The listing builds one solid part. Answer for the finished solid, in the listing's coordinates (mm). Face numbers are marked on the shaded views. A direction names the side the tool comes from. Coordinates: 2 decimals unless noted, no trailing zeros. Order: outer loops, then holes, each group sorted by start corner. A loop starts at its lowest first (then second) coordinate and runs counter-clockwise, first axis right, second up. Notation, with made-up numbers: (37, -9.5) -> (78, -9.5) arc R6 ccw to (78, 0.5) -> close; hole circle Ø8 at (-2, -28.75). An arc over 180 degrees is marked (long way). Return JSON: item names as keys, results as strings.
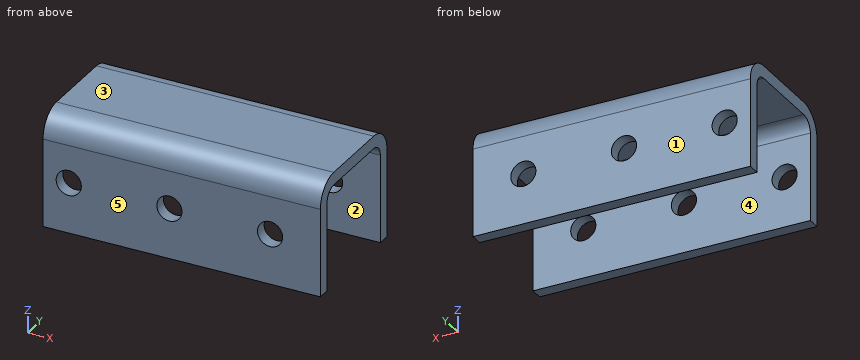
```python
from build123d import *

# Parameters (mm, degrees)
SKETCH1_W          = 889
SKETCH1_H          = 31.75
EXTRUDE1_DEPTH     = 28.575
EXTRUDE2_REACH     = 891
SKETCH2_W          = 25.4
SKETCH2_H          = 25.4
HOLE1_D            = 6.35
HOLE1_DEPTH        = 3.175
LPATTERN1_COUNT    = 35
LPATTERN1_PITCH    = 25.4
HOLE2_D            = 9.652
HOLE2_DEPTH        = 3.175
LPATTERN2_COUNT    = 12
LPATTERN2_PITCH    = 25.4
HOLE3_D            = 9.652
HOLE3_DEPTH        = 3.175
HOLE4_D            = 9.652
HOLE4_DEPTH        = 3.175
LPATTERN3_COUNT    = 12
LPATTERN3_PITCH    = 25.4
HOLE5_D            = 3.175
HOLE5_DEPTH        = 3.175
HOLE6_D            = 6.35
HOLE6_DEPTH        = 3.175
LPATTERN4_COUNT    = 35
LPATTERN4_PITCH    = 25.4
FILLET1_R          = 3.175
FILLET2_R          = 3.175
FILLET3_R          = 6.35
FILLET4_R          = 6.35
SKETCH16_W         = 145.760071232
SKETCH16_H         = 71.504803879
CUT_EXTRUDE2_DEPTH = 75
SKETCH17_W         = 473.628565651
SKETCH17_H         = 66.908943447
CUT_EXTRUDE3_DEPTH = 186
SKETCH18_W         = 373.094897193
SKETCH18_H         = 93.915816603
CUT_EXTRUDE4_DEPTH = 186


with BuildPart() as part:
    # Sketch1 → Extrude1 (new body)
    with BuildSketch(Plane.XY.offset(3.175)):
        with Locations((428.480011997, 8.672957166)):
            Rectangle(SKETCH1_W, SKETCH1_H)
    extrude(amount=-EXTRUDE1_DEPTH)

    # Sketch2 → Extrude2 (cut, up to next)
    with BuildSketch(Plane.ZY.offset(16.019988003), mode=Mode.PRIVATE) as extrude2_sk1:
        with Locations((-12.7, 8.672957166)):
            Rectangle(SKETCH2_W, SKETCH2_H)
    extrude2_tool1 = extrude(extrude2_sk1.sketch, amount=-EXTRUDE2_REACH, mode=Mode.PRIVATE) & part.part
    add(extrude2_tool1.solids().sort_by_distance((-16.019988, 8.672957, -12.7))[0], mode=Mode.SUBTRACT)

    # Hole1
    with Locations(Plane(origin=(0, 24.547957166, 0), x_dir=(-1, 0, 0), z_dir=(0, 1, 0))):
        with Locations((3.319988003, -12.7)):
            hole1 = Hole(HOLE1_D / 2, depth=HOLE1_DEPTH)

    # LPattern1: Hole1 ×35
    with Locations(*[(i * LPATTERN1_PITCH, 0, 0) for i in range(1, LPATTERN1_COUNT)]):
        add(hole1, mode=Mode.SUBTRACT)

    # Hole2
    with Locations(Plane.XY.offset(3.175)):
        with Locations((66.530011997, 10.577957166)):
            hole2 = Hole(HOLE2_D / 2, depth=HOLE2_DEPTH)

    # LPattern2: Hole2 ×12, 8 skipped
    with Locations(*[(i * LPATTERN2_PITCH, 0, 0) for i in range(1, LPATTERN2_COUNT) if i not in (2, 3, 4, 5, 6, 7, 8, 9)]):
        add(hole2, mode=Mode.SUBTRACT)

    # Hole3
    with Locations(Plane.XY.offset(3.175)):
        with Locations((428.480011997, 6.767957166)):
            Hole(HOLE3_D / 2, depth=HOLE3_DEPTH)

    # Hole4
    with Locations(Plane.XY.offset(3.175)):
        with Locations((511.030011997, 10.577957166)):
            hole4 = Hole(HOLE4_D / 2, depth=HOLE4_DEPTH)

    # LPattern3: Hole4 ×12, 8 skipped
    with Locations(*[(i * LPATTERN3_PITCH, 0, 0) for i in range(1, LPATTERN3_COUNT) if i not in (2, 3, 4, 5, 6, 7, 8, 9)]):
        add(hole4, mode=Mode.SUBTRACT)

    # Hole5
    with Locations(Plane.XY.offset(3.175)):
        with Locations((669.780011997, 8.672957166)):
            Hole(HOLE5_D / 2, depth=HOLE5_DEPTH)

    # Hole6
    with Locations(Plane(origin=(0, -4.027042834, 0), x_dir=(-1, 0, 0), z_dir=(0, 1, 0))):
        with Locations((3.319988003, -12.7)):
            hole6 = Hole(HOLE6_D / 2, depth=HOLE6_DEPTH)

    # LPattern4: Hole6 ×35
    with Locations(*[(i * LPATTERN4_PITCH, 0, 0) for i in range(1, LPATTERN4_COUNT)]):
        add(hole6, mode=Mode.SUBTRACT)

    # Fillet1
    fillet1_edges = [part.edges().sort_by_distance(p)[0] for p in [
        (428.480011997, 21.372957166, 0),
    ]]
    fillet(fillet1_edges, radius=FILLET1_R)

    # Fillet2
    fillet2_edges = [part.edges().sort_by_distance(p)[0] for p in [
        (428.480011997, -4.027042834, 0),
    ]]
    fillet(fillet2_edges, radius=FILLET2_R)

    # Fillet3
    fillet3_edges = [part.edges().sort_by_distance(p)[0] for p in [
        (428.480011997, -7.202042834, 3.175),
    ]]
    fillet(fillet3_edges, radius=FILLET3_R)

    # Fillet4
    fillet4_edges = [part.edges().sort_by_distance(p)[0] for p in [
        (428.480011997, 24.547957166, 3.175),
    ]]
    fillet(fillet4_edges, radius=FILLET4_R)

    # Sketch16 → Cut-Extrude2 (cut)
    with BuildSketch(Plane(origin=(0, 24.547957166, 0), x_dir=(1, 0, 0), z_dir=(0, 1, 0))):
        with Locations((40.099976381, -10.352401939)):
            Rectangle(SKETCH16_W, SKETCH16_H)
    extrude(amount=-CUT_EXTRUDE2_DEPTH, mode=Mode.SUBTRACT)

    # Sketch17 → Cut-Extrude3 (cut)
    with BuildSketch(Plane(origin=(0, 24.547957166, 0), x_dir=(1, 0, 0), z_dir=(0, 1, 0))):
        with Locations((288.165729172, -8.054471723)):
            Rectangle(SKETCH17_W, SKETCH17_H)
    extrude(amount=-CUT_EXTRUDE3_DEPTH, mode=Mode.SUBTRACT)

    # Sketch18 → Cut-Extrude4 (cut)
    with BuildSketch(Plane(origin=(0, 24.547957166, 0), x_dir=(1, 0, 0), z_dir=(0, 1, 0))):
        with Locations((616.432563401, -21.557908301)):
            Rectangle(SKETCH18_W, SKETCH18_H)
    extrude(amount=-CUT_EXTRUDE4_DEPTH, mode=Mode.SUBTRACT)


solid = part.part
```
Item 1: Determine the mould class of the marked faces 1, 2 and 3 for opening direction Y: pulls with the +Y half, pulls with the -Y half, needs draft (parallel to the pull), parting line crosses it, or undercut.
Answer list:
{"face 1": "pulls with the +Y half", "face 2": "undercut", "face 3": "needs draft"}
Item 2: Which of the six approach directions +Z, -Z, +X, -X, +Y, -Y give full straight-line access (tool end or side, diameter ignored) to the marked faces 4 and 5?
Answer list:
{"face 4": "-Z, +X, -X", "face 5": "+Z, -Z, +X, -X, -Y"}
Item 3: The part is cut by section B-B on z = -12.7. Count the separate pieces of the cut face and the enclosed holes in it, plus the area to 3 significant figures.
Answer list:
{"separate pieces": "8", "enclosed holes": "0", "area": "324 mm2"}
Item 4: The part is cut by section D-D on x = 861.5. Determine the outline of the cut face in (y, z) (3 decimals).
Answer list:
{"outline": "(-7.202, -25.4) -> (-4.027, -25.4) -> (-4.027, -15.631) -> (-7.202, -15.631) -> close; (-7.202, -9.769) -> (-4.027, -9.769) -> (-4.027, -3.175) arc R3.175 cw to (-0.852, 0) -> (18.198, 0) arc R3.175 cw to (21.373, -3.175) -> (21.373, -9.769) -> (24.548, -9.769) -> (24.548, -3.175) arc R6.35 ccw to (18.198, 3.175) -> (-0.852, 3.175) arc R6.35 ccw to (-7.202, -3.175) -> close; (21.373, -25.4) -> (24.548, -25.4) -> (24.548, -15.631) -> (21.373, -15.631) -> close"}
Item 5: The part is cut by section C-C on y = 4.5. Determine the outline of the cut face in (x, z) (3 decimals), plus the area to 3 significant figures.
Answer list:
{"outline": "(802.98, 0) -> (872.98, 0) -> (872.98, 3.175) -> (802.98, 3.175) -> close", "area": "222 mm2"}
Item 6: The part is cut by section A-A on x = 810.5. Determine the outline of the cut face in (y, z) (3 decimals), plus the area to 3 significant figures.
Answer list:
{"outline": "(-7.202, -25.4) -> (-4.027, -25.4) -> (-4.027, -15.707) -> (-7.202, -15.707) -> close; (-7.202, -9.693) -> (-4.027, -9.693) -> (-4.027, -3.175) arc R3.175 cw to (-0.852, 0) -> (18.198, 0) arc R3.175 cw to (21.373, -3.175) -> (21.373, -9.693) -> (24.548, -9.693) -> (24.548, -3.175) arc R6.35 ccw to (18.198, 3.175) -> (-0.852, 3.175) arc R6.35 ccw to (-7.202, -3.175) -> close; (21.373, -25.4) -> (24.548, -25.4) -> (24.548, -15.707) -> (21.373, -15.707) -> close", "area": "211 mm2"}
Item 7: Flat-ended cylindrical pins translate along their axes: pin 1 (8.5 mm diameter, centred on x = 860.28, z = -12.7, fed in from -Y); pin 2 (5 mm diameter, centred on x = 852, y = -1, fed in from -Z); pin 3 (5.5 mm diameter, centred on x = 826, y = 7, fed in from -Z). Find the tip coordinate at first contact, or state that the pin passes through.
Answer list:
{"pin 1": "y = -7.2", "pin 2": "z = -1.42", "pin 3": "z = 0"}
Item 8: Find the intervals of material crossed by probe 1 along Y at (x, z) = (822, -22); probe 2 along Z at (x, y) = (808, 16) (3 decimals); probe 3 along Y at (x, z) = (834, -1.25), in increasing order.
Answer list:
{"probe 1": "-7.2 to -4.03, 21.37 to 24.55", "probe 2": "0 to 3.175", "probe 3": "-6.9 to -3.38, 20.72 to 24.25"}
